from build123d import *

# Parameters (mm, degrees)
F0_W      = 89
F0_H      = 18.8
F1_DEPTH  = 3
F2_W      = 12
F2_H      = 6
F3_W      = 12
F3_H      = 6
F4_DEPTH  = 8.5
F5_R      = 1.5
F6_DEPTH  = 89.001
F7_R      = 1.5
F8_R      = 1.5
F9_DEPTH  = 15
F10_W     = 45
F10_H     = 9
F11_DEPTH = 25


with BuildPart() as f1:
    # F0 (on Top) → F1 (new body)
    with BuildSketch(Plane.XY):
        Rectangle(F0_W, F0_H)
    extrude(amount=F1_DEPTH)

    # F2 (on face) + F3 (on face) → F4 (join)
    with BuildSketch(Plane.XY.offset(3)):
        with Locations((38.5, 6.4)):
            Rectangle(F2_W, F2_H)
    with BuildSketch(Plane.XY.offset(3)):
        with Locations((-38.5, 6.4)):
            Rectangle(F3_W, F3_H)
    extrude(amount=F4_DEPTH)

    # F5 (on face) → F6 (cut, through all)
    with BuildSketch(Plane(origin=(-44.5, 0, 0), x_dir=(0, -1, 0), z_dir=(-1, 0, 0))):
        with Locations((-6.4, 7.5)):
            Circle(F5_R)
    extrude(amount=-F6_DEPTH, mode=Mode.SUBTRACT)

    # F7 (on face) + F8 (on face) → F9 (cut)
    with BuildSketch(Plane.XY.offset(3)):
        with Locations((21.5, -4.4)):
            Circle(F7_R)
    with BuildSketch(Plane.XY.offset(3)):
        with Locations((-34.5, -4.4)):
            Circle(F8_R)
    extrude(amount=-F9_DEPTH, mode=Mode.SUBTRACT)

    # F10 (on face) → F11 (cut)
    with BuildSketch(Plane(origin=(0, 0, 0), x_dir=(1, 0, 0), z_dir=(0, 0, -1))):
        with Locations((-5.5, 4.9)):
            Rectangle(F10_W, F10_H)
    extrude(amount=-F11_DEPTH, mode=Mode.SUBTRACT)


solid = f1.part
Geometry check sheet. Reference: the model listing, model coordinates, mm. A direction names the side the tool comes from. Give positions to 0.01 mm unless a question says otherwise; leave off trailing zeros. Write each loop counter-clockwise with the first axis right and the second up, starting at its lowest first coordinate (ties: lowest second). Pieces come first, ordered by that corner, then holes. Notation, with made-up numbers: (42.5, 53.5) - (101.5, 53.5) arc R22 cw to (101.5, 65.5) - close; hole circle Ø5 at (29.25, -17). An arc over 180 degrees is marked (long way). Put each result on its own line as item: value.
1. Thickness scan on line 1 (Z direction, x = 40.5, y = 6.4); line 2 (X direction, y = -3.5, z = 1.25); line 3 (Y direction, x = 38.5, z = 9.5). Record the ranges inside material, lowest first.
Ans:
line 1: z = 0 to 6, 9 to 11.5
line 2: x = -44.5 to -35.7, -33.3 to -28, 17 to 20.3, 22.7 to 44.5
line 3: y = 3.4 to 9.4
2. Sectioned sample at D-D, the plane y = 6.4. Enter the section's corners in (x, z), plus the area to 3 significant figures.
Ans:
outline: (-44.5, 0) - (44.5, 0) - (44.5, 6) - (32.5, 6) - (32.5, 3) - (-32.5, 3) - (-32.5, 6) - (-44.5, 6) - close; (-44.5, 9) - (-32.5, 9) - (-32.5, 11.5) - (-44.5, 11.5) - close; (32.5, 9) - (44.5, 9) - (44.5, 11.5) - (32.5, 11.5) - close
area: 399 mm²
3. Sectioned sample at C-C, the plane z = 1.75. Enter the section's corners in (x, y), plus the area to 3 significant figures.
Ans:
outline: (-44.5, -9.4) - (-28, -9.4) - (-28, -0.4) - (17, -0.4) - (17, -9.4) - (44.5, -9.4) - (44.5, 9.4) - (-44.5, 9.4) - close; hole circle Ø3 at (-34.5, -4.4); hole circle Ø3 at (21.5, -4.4)
area: 1,250 mm²
4. Sectioned sample at B-B, the plane x = 21.5. Enter the section's corners in (y, z), plus the area to 3 significant figures.
Ans:
outline: (-9.4, 0) - (-5.9, 0) - (-5.9, 3) - (-9.4, 3) - close; (-2.9, 0) - (9.4, 0) - (9.4, 3) - (-2.9, 3) - close
area: 47.4 mm²
5. Go/stop test with flat-tipped pins: pin 1 (0.9 mm diameter, centred on x = -4.5, z = 1.5, fed in from -Y); pin 2 (2.5 mm diameter, centred on x = -35.5, z = 7.5, fed in from -Y); pin 3 (4 mm diameter, centred on x = -34.5, y = -4.4, fed in from +Z). Record where each tip stops, or that it passes through.
Ans:
pin 1: stops at y = -0.4
pin 2: stops at y = 3.4
pin 3: stops at z = 3
6. Set-up check for faces 5 (the flat face through (-32.5, 5, 6)), 6 (the flat face through (-28, -5, 1)), 7 (the flat face through (-39, 3.4, 7)), 8 (the cylindrical face through (-38.58, 5.71, 6.17)): record each of +Z, -Z, +X, -X, +Y, -Y from which the full face is reachable in a straight line by a thin tool's end or side.
Ans:
face 5: +Z, +Y, -Y
face 6: +Z, -Z, -Y
face 7: +Z, +X, -X, -Y
face 8: +X, -X
7. Sectioned sample at A-A, the plane y = -4.4. Enter the section's corners in (x, z).
Ans:
outline: (-44.5, 0) - (-36, 0) - (-36, 3) - (-44.5, 3) - close; (-33, 0) - (-28, 0) - (-28, 3) - (-33, 3) - close; (17, 0) - (20, 0) - (20, 3) - (17, 3) - close; (23, 0) - (44.5, 0) - (44.5, 3) - (23, 3) - close
8. Draft check along Z on faces 1 (the flat face through (-39, 6, 11.5)), 2 (the flat face through (-6, -0.4, 1)), 3 (the flat face through (-1, 2, 0)), 4 (the cylindrical face through (38.42, 5.71, 6.17)). Enter one of: +Z half, -Z half, draft (parallel to the pull), parting line (faces both ways), or undercut.
Ans:
face 1: +Z half
face 2: draft
face 3: -Z half
face 4: undercut
